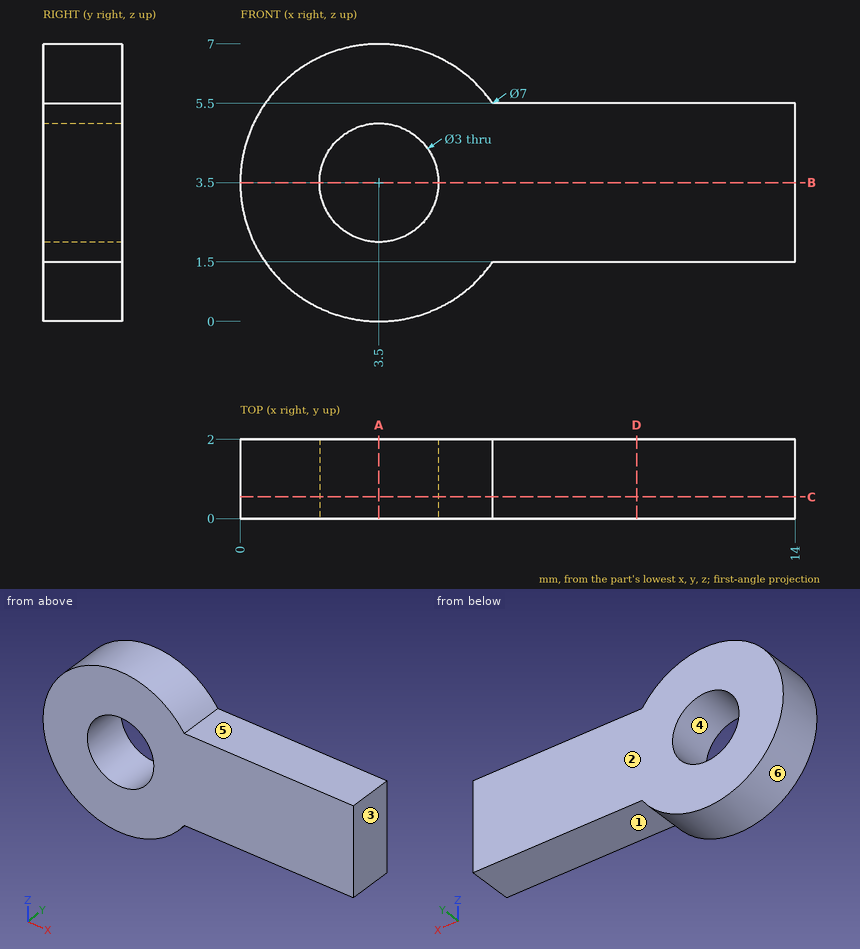
Verification items for this drawing (mm, ordinates from the low corner). A direction names the side the tool comes from. Give positions to 0.01 mm unless a question says otherwise; leave off trailing zeros. Loops run counter-clockwise (first coordinate to the right, second up) from the corner with the lowest first, then second, coordinate; pieces in that order, holes last. Notation, with made-up numbers: M 50.5,55 L 90.5,55 A14 cw 90.5,70 Z; hole C 1.5,42 d4. An arc over 180 degrees is marked long. Answer in a Markdown table with one row per item.
1) Tool access check on the marked faces 1 and 2. Record the directions out of +Z, -Z, +X, -X, +Y, -Y that give a thin tool (end or side, any length) a straight path to the whole face; none if there is none.
Solutions:
| item | result |
|---|---|
| face 1 | -Z, +X, +Y, -Y |
| face 2 | +Z, -Z, +X, -X, +Y |
2) Cross-section at C-C (y = 0.55). Enter the section's corners in (x, z).
Solutions:
| item | result |
|---|---|
| outline | M 6.37,1.5 L 14,1.5 L 14,5.5 L 6.37,5.5 A3.5 ccw long Z; hole C 3.5,3.5 d3 |
3) Mould release check, pull along X, two halves, no side actions. Record for the marked faces 3, 4, 5 and 6: released by +X, released by -X, zero draft, split by the parting line, or undercut.
Solutions:
| item | result |
|---|---|
| face 3 | released by +X |
| face 4 | undercut |
| face 5 | zero draft |
| face 6 | split by the parting line |
4) Thickness scan on line 1 (X direction, y = 1.55, z = 3.5); line 2 (Z direction, x = 13.25, y = 0.8); line 3 (Z direction, x = 3.25, y = 0.25). Record the ranges inside material, lowest first.
Solutions:
| item | result |
|---|---|
| line 1 | x = 0 to 2, 5 to 14 |
| line 2 | z = 1.5 to 5.5 |
| line 3 | z = 0.01 to 2.02, 4.98 to 6.99 |
5) Cross-section at A-A (x = 3.5). Enter the section's corners in (y, z), plus the area to 3 significant figures.
Solutions:
| item | result |
|---|---|
| outline | M 0,0 L 2,0 L 2,2 L 0,2 Z; M 0,5 L 2,5 L 2,7 L 0,7 Z |
| area | 8.00 mm^2 |
6) Cross-section at D-D (x = 10). Enter the section's corners in (y, z), plus the area to 3 significant figures.
Solutions:
| item | result |
|---|---|
| outline | M 0,1.5 L 2,1.5 L 2,5.5 L 0,5.5 Z |
| area | 8.00 mm^2 |
7) Depth check by flat-ended pin: pin 1 (1 mm diameter, centred on x = 8.5, y = 1, fed in from -Z); pin 2 (4 mm diameter, centred on x = 2.5, z = 3.5, fed in from +Y); pin 3 (2.5 mm diameter, centred on x = 3.5, z = 3.5, fed in from +Y); pin 4 (1 mm diameter, centred on x = 10.5, y = 1, fed in from +Z). Enter the tip coordinate at first touch or a pass-through.
Solutions:
| item | result |
|---|---|
| pin 1 | stops at z = 1.5 |
| pin 2 | stops at y = 2 |
| pin 3 | passes through |
| pin 4 | stops at z = 5.5 |
8) Cross-section at B-B (z = 3.5). Enter the section's corners in (x, y).
Solutions:
| item | result |
|---|---|
| outline | M 0,0 L 2,0 L 2,2 L 0,2 Z; M 5,0 L 14,0 L 14,2 L 5,2 Z |
